from build123d import *

# Parameters (mm, degrees)
SKETCH1_R           = 2
SKETCH1_R_2         = 11.9
BOSS_EXTRUDE1_DEPTH = 6.2
CUT_EXTRUDE1_DEPTH  = 1


with BuildPart() as part:
    # Sketch1 → Boss-Extrude1 (new body)
    with BuildSketch(Plane(origin=(0, 0, 0), x_dir=(1, 0, 0), z_dir=(0, 1, 0))):
        Polygon((-30, -6.2), (0, -36.2), (0, -73.8), (6.2, -73.8), (6.2, -80), (12.4, -80), (12.4, -73.8), (18.6, -73.8), (18.6, -80), (24.8, -80), (24.8, -73.8), (56.4, -73.8), (56.4, -80), (62.6, -80), (62.6, -73.8), (68.8, -73.8), (68.8, -80), (75, -80), (75, -73.8), (81.2, -73.8), (81.2, -67.6), (75, -67.6), (75, -61.4), (81.2, -61.4), (81.2, -55.2), (75, -55.2), (75, -24.8), (81.2, -24.8), (81.2, -18.6), (75, -18.6), (75, -12.4), (81.2, -12.4), (81.2, -6.2), (75, -6.2), (75, 0), (68.8, 0), (68.8, -6.2), (62.6, -6.2), (62.6, 0), (56.4, 0), (56.4, -6.2), (24.8, -6.2), (24.8, 0), (18.6, 0), (18.6, -6.2), (12.4, -6.2), (12.4, 0), (6.2, 0), (6.2, -6.2), align=None)
        with Locations((53.744267305, -31.89475279)):
            Circle(SKETCH1_R, mode=Mode.SUBTRACT)
        with Locations((21.41882184, -46.37677641)):
            Circle(SKETCH1_R, mode=Mode.SUBTRACT)
        with Locations((60.62, -56.23)):
            Circle(SKETCH1_R_2, mode=Mode.SUBTRACT)
    extrude(amount=BOSS_EXTRUDE1_DEPTH)

    # Sketch2 → Cut-Extrude1 (cut)
    with BuildSketch(Plane(origin=(0, 6.2, 0), x_dir=(1, 0, 0), z_dir=(0, 1, 0))):
        with BuildLine():
            Line((12.966892289, -13.0509751), (12.966892289, -13.376616125))
            Line((12.966892289, -13.376616125), (11.886934356, -13.376616125))
            Line((11.886934356, -13.376616125), (11.715845614, -14.211707271))
            add(Edge.make_bspline(
                [(11.715845614, -14.211707271), (11.749460586, -14.202426953), (11.814584277, -14.184447805), (11.910705008, -14.164485427), (12.001956507, -14.152451775), (12.061170593, -14.150808657), (12.08982398, -14.150013561)],
                knots=[0, 0, 0, 0, 0.000104595, 0.000202637, 0.000294305, 0.000380252, 0.000380252, 0.000380252, 0.000380252], degree=3))
            add(Edge.make_bspline(
                [(12.08982398, -14.150013561), (12.125278515, -14.150780946), (12.19499099, -14.152289816), (12.296989177, -14.166778565), (12.394355445, -14.189584059), (12.486886166, -14.221443389), (12.574752523, -14.262182933), (12.657146096, -14.313073593), (12.735303632, -14.372521686), (12.807822985, -14.440870376), (12.873612893, -14.516092128), (12.931457755, -14.596971054), (12.980590962, -14.682721147), (13.02010679, -14.7741617), (13.05166115, -14.870281789), (13.072663317, -14.972092774), (13.086648474, -15.078634998), (13.088210925, -15.151482715), (13.089007673, -15.188630348)],
                knots=[0, 0, 0, 0, 0.000106308, 0.000209029, 0.000308378, 0.000405929, 0.000502102, 0.000598312, 0.00069588, 0.000796219, 0.000896736, 0.000995218, 0.001094066, 0.001192613, 0.001293582, 0.001396995, 0.001504047, 0.001615439, 0.001615439, 0.001615439, 0.001615439], degree=3))
            add(Edge.make_bspline(
                [(13.089007673, -15.188630348), (13.088404355, -15.214504077), (13.087205872, -15.265901873), (13.081111153, -15.342232683), (13.069376611, -15.416947539), (13.053621604, -15.490056352), (13.03317241, -15.561420711), (13.00841734, -15.631244882), (12.978122372, -15.699094276), (12.944892482, -15.765610884), (12.907476034, -15.829290958), (12.865948388, -15.888843968), (12.822073978, -15.94516328), (12.774865007, -15.997644881), (12.723882676, -16.045943904), (12.66974442, -16.090346988), (12.612882239, -16.131605052), (12.552416412, -16.168043343), (12.489694303, -16.201574025), (12.423810134, -16.229081805), (12.356263642, -16.253674927), (12.286082647, -16.273277856), (12.213426117, -16.288638102), (12.138174285, -16.299070789), (12.06072182, -16.306669415), (12.008220916, -16.307145081), (11.981700983, -16.307385356)],
                knots=[0, 0, 0, 0, 7.7636e-05, 0.000154223, 0.000229512, 0.000304362, 0.000378447, 0.000452077, 0.000526407, 0.000601214, 0.00067506, 0.000747747, 0.00081887, 0.000889121, 0.000959302, 0.001029336, 0.001099058, 0.00116985, 0.001240974, 0.00131221, 0.00138383, 0.001456517, 0.001530612, 0.001606437, 0.001684346, 0.001763871, 0.001763871, 0.001763871, 0.001763871], degree=3))
            add(Edge.make_bspline(
                [(11.981700983, -16.307385356), (11.950065119, -16.306758667), (11.887825294, -16.305525731), (11.796638779, -16.292627534), (11.708904816, -16.274154553), (11.625329653, -16.246363079), (11.545164292, -16.211540319), (11.469487969, -16.167529221), (11.396367015, -16.11765532), (11.328773953, -16.058799571), (11.266039479, -15.994468916), (11.209881432, -15.924657342), (11.159867401, -15.850517062), (11.116798302, -15.771688023), (11.080060812, -15.688377355), (11.051200072, -15.600272919), (11.027906136, -15.507835058), (11.018051462, -15.444195802), (11.013046135, -15.411872536)],
                knots=[0, 0, 0, 0, 9.4843e-05, 0.000186593, 0.000275792, 0.000363484, 0.000450342, 0.000537514, 0.000625728, 0.000715478, 0.000805885, 0.000894984, 0.00098389, 0.001073836, 0.001164117, 0.001256635, 0.001351658, 0.001449737, 0.001449737, 0.001449737, 0.001449737], degree=3))
            Line((11.013046135, -15.411872536), (11.297982032, -15.411872536))
            add(Edge.make_bspline(
                [(11.297982032, -15.411872536), (11.304992938, -15.442149746), (11.318468288, -15.500344226), (11.34804636, -15.582106228), (11.384210404, -15.654967238), (11.42721292, -15.719891075), (11.478511877, -15.776504951), (11.537049287, -15.826957571), (11.602679007, -15.872473581), (11.675607151, -15.910412806), (11.75254473, -15.942769461), (11.833069271, -15.964315641), (11.914988214, -15.979465737), (11.970395021, -15.980982263), (11.998237441, -15.981744331)],
                knots=[0, 0, 0, 0, 9.3172e-05, 0.000179081, 0.000260145, 0.000336703, 0.000411917, 0.000488562, 0.000568128, 0.000650923, 0.00073478, 0.000817953, 0.000900557, 0.000983994, 0.000983994, 0.000983994, 0.000983994], degree=3))
            add(Edge.make_bspline(
                [(11.998237441, -15.981744331), (12.02541403, -15.980999768), (12.078924956, -15.979533718), (12.157675285, -15.968249757), (12.233705535, -15.950871103), (12.306265495, -15.924863448), (12.376624891, -15.893254311), (12.443003954, -15.852691349), (12.507322993, -15.806009761), (12.5675828, -15.752527675), (12.622772872, -15.693590881), (12.671537353, -15.63056496), (12.71215641, -15.563330392), (12.746386638, -15.493051175), (12.772379273, -15.418957055), (12.790922163, -15.341395275), (12.801810652, -15.260174257), (12.803308508, -15.204775669), (12.804071776, -15.176546013)],
                knots=[0, 0, 0, 0, 8.15e-05, 0.000160473, 0.000238226, 0.000315066, 0.000391338, 0.000469218, 0.000547964, 0.000629516, 0.000710512, 0.000789892, 0.000868102, 0.000945761, 0.001024012, 0.00110315, 0.001184644, 0.001269321, 0.001269321, 0.001269321, 0.001269321], degree=3))
            add(Edge.make_bspline(
                [(12.804071776, -15.176546013), (12.803474441, -15.151077296), (12.802305243, -15.101225905), (12.792752511, -15.028292339), (12.776136401, -14.959283222), (12.75307331, -14.89386531), (12.723791185, -14.831976902), (12.688007744, -14.773554125), (12.645051448, -14.719367005), (12.595982377, -14.669390189), (12.542226869, -14.623266624), (12.482860045, -14.583947345), (12.419124254, -14.550869363), (12.351787403, -14.522323393), (12.279247817, -14.501821288), (12.202942015, -14.486428992), (12.122046001, -14.477525056), (12.066736877, -14.476289629), (12.038306552, -14.475654587)],
                knots=[0, 0, 0, 0, 7.6388e-05, 0.000149519, 0.000220172, 0.000288967, 0.000357247, 0.000425206, 0.000494043, 0.000564207, 0.000635056, 0.000706145, 0.000777268, 0.000850264, 0.000925136, 0.001002969, 0.001083601, 0.001168886, 0.001168886, 0.001168886, 0.001168886], degree=3))
            add(Edge.make_bspline(
                [(12.038306552, -14.475654587), (12.013696738, -14.476181266), (11.962883715, -14.477268725), (11.884939437, -14.485275618), (11.803031945, -14.498192693), (11.717475224, -14.515960217), (11.628012335, -14.539211265), (11.534832071, -14.567073705), (11.437738515, -14.600385804), (11.372317437, -14.625542884), (11.338687161, -14.6384751)],
                knots=[0, 0, 0, 0, 7.3822e-05, 0.000152423, 0.000234822, 0.000322511, 0.00041445, 0.000512043, 0.000614219, 0.000722306, 0.000722306, 0.000722306, 0.000722306], degree=3))
            Line((11.338687161, -14.6384751), (11.664328186, -13.0509751))
            Line((11.664328186, -13.0509751), (12.966892289, -13.0509751))
        make_face()
        Polygon((15.147796736, -12.969564843), (15.20567434, -12.969564843), (15.20567434, -15.167641766), (15.572020494, -15.167641766), (15.572020494, -15.493282792), (15.20567434, -15.493282792), (15.20567434, -16.2259751), (14.920738443, -16.2259751), (14.920738443, -15.493282792), (13.414648699, -15.493282792), align=None)
        Polygon((14.920738443, -15.167641766), (14.920738443, -13.788755549), (13.974344212, -15.167641766), align=None, mode=Mode.SUBTRACT)
    extrude(amount=-CUT_EXTRUDE1_DEPTH, mode=Mode.SUBTRACT)


solid = part.part
Input: part model. Units: mm. Frame: model coordinates. A direction names the side the tool comes from. Coordinates: 2 decimals unless noted, no trailing zeros. Order: outer loops, then holes, each group sorted by start corner. A loop starts at its lowest first (then second) coordinate and runs counter-clockwise, first axis right, second up. Notation, with made-up numbers: M 8,-12 L 46,-12 A30 cw 46,22 Z; hole C 39.5,18 d10. An arc over 180 degrees is marked long. Write item = value, one per line. Start each with the question number.
(1) Section A-A on x = 60.62. Output: boundary loops of the cut face in (y, z), and give its area (3 significant figures).
(2) Line query: line 1 along X through (y, z) = (4.25, 76.5); line 2 along Z through (x, y) = (60.62, 1.75); line 3 along X through (y, z) = (2.75, 56.23). Output: solid intervals per line, ascending. Write a range as [from, to].
(3) Section C-C on y = 2. Give the number of separate pieces and of enclosed holes in the cut face, and give its area (3 significant figures).
(4) Pull-direction query (X, two-part tool) for faces 1 (the flat face through (78, 3, 67.6)), 2 (the flat face through (12.21, 5.2, 14.31)), 3 (the flat face through (75, 3, 77)); classes: released by +X, released by -X, zero draft, split by the parting line, or undercut.
(5) Section D-D on x = -13.5. Output: boundary loops of the cut face in (y, z), and give its area (3 significant figures).
(6) First-contact query: P1, Ø1.9, axis at x = 78.5, y = 3, coming from the -Z side; P2, Ø1.9, axis at y = 3, z = 4, coming from the +X side; P3, Ø3, axis at y = 3.5, z = 76.5, coming from the -X side. Flat tips, straight axial feed; report the tip coordinate or a pass-through.
(7) Reachability of faces 4 (the flat face through (18.6, 3, 3)), 5 (the flat face through (78, 3, 6.2)), 6 (the flat face through (75, 3, 16)), 7 (the flat face through (0, 3, 55)), 8 (the flat face through (40, 3, 73.8)) from +Z, -Z, +X, -X, +Y, -Y: full face, straight path, thin tool, end or side. Return the list, or none.
(8) Section B-B on z = 64. Output: boundary loops of the cut face in (x, y).
Result set:
q1.outline = M 0,0 L 6.2,0 L 6.2,44.33 L 0,44.33 Z; M 0,68.13 L 6.2,68.13 L 6.2,80 L 0,80 Z
q1.area = 348 mm²
q2.line_1 = [6.2, 12.4], [18.6, 24.8], [56.4, 62.6], [68.8, 75]
q2.line_2 = [0, 44.33], [68.13, 80]
q2.line_3 = [0, 48.72], [72.52, 81.2]
q3.separate_pieces = 1
q3.enclosed_holes = 3
q3.area = 5,510 mm²
q4.face_1 = zero draft
q4.face_2 = undercut
q4.face_3 = released by +X
q5.outline = M 0,6.2 L 6.2,6.2 L 6.2,22.7 L 0,22.7 Z
q5.area = 102 mm²
q6.P1 = 6.2
q6.P2 = 75
q6.P3 = 6.2
q7.face_4 = -Z, +Y, -Y
q7.face_5 = -Z, +X, +Y, -Y
q7.face_6 = +X, +Y, -Y
q7.face_7 = +Z, -X, +Y, -Y
q7.face_8 = +Z, +Y, -Y
q8.outline = M 0,0 L 51.61,0 L 51.61,6.2 L 0,6.2 Z; M 69.63,0 L 75,0 L 75,6.2 L 69.63,6.2 Z
